Build history of the part. All positions in model axes, mm. A direction names the side the tool comes from. Round coordinates to 2 decimals unless told otherwise and drop trailing zeros. Order: outer loops, then holes, each group sorted by start corner. A loop starts at its lowest first (then second) coordinate and runs counter-clockwise, first axis right, second up. Notation, with made-up numbers: (0, -38.5) -> (31, -38.5) arc R26 ccw to (31, -2.5) -> close; hole circle Ø4 at (-38, 63.25). An arc over 180 degrees is marked (long way). Answer as a JSON object with one key per item and string values.
from build123d import *

# Parameters (mm, degrees)
SKETCH_3_W          = 100
SKETCH_3_H          = 40
EXTRUDE_1_DEPTH     = 10
EXTRUDE_3_DEPTH     = 10
SKETCH_6_R          = 12.5
CUT_EXTRUDE_1_DEPTH = 5
SKETCH_8_R          = 6
CUT_EXTRUDE_2_DEPTH = 5
SKETCH_9_W          = 30
SKETCH_9_H          = 5
CUT_EXTRUDE_4_DEPTH = 85.409715081
FILLET_1_R          = 8
SKETCH_12_R         = 4
CUT_EXTRUDE_6_DEPTH = 71.178344238
FILLET_2_R          = 3


with BuildPart() as part:
    # Эскиз3 → Бобышка-Вытянуть1 (new body)
    with BuildSketch(Plane(origin=(0, 0, 0), x_dir=(1, 0, 0), z_dir=(0, 1, 0))):
        Rectangle(SKETCH_3_W, SKETCH_3_H)
    extrude(amount=EXTRUDE_1_DEPTH)

    # Эскиз4 → Бобышка-Вытянуть3 (add)
    with BuildSketch(Plane(origin=(0, 0, -20), x_dir=(-1, 0, 0), z_dir=(0, 0, -1))):
        with BuildLine():
            Line((-20, 0), (-20, 35))
            ThreePointArc((-20, 35), (0, 55), (20, 35))
            Line((20, 35), (20, 0))
            Line((20, 0), (-20, 0))
        make_face()
    extrude(amount=-EXTRUDE_3_DEPTH)

    # Эскиз6 → Вырез-Вытянуть1 (cut)
    with BuildSketch(Plane(origin=(0, 0, -20), x_dir=(-1, 0, 0), z_dir=(0, 0, -1))):
        with Locations((0, 35)):
            Circle(SKETCH_6_R)
    extrude(amount=-CUT_EXTRUDE_1_DEPTH, mode=Mode.SUBTRACT)

    # Эскиз8 → Вырез-Вытянуть2 (cut)
    with BuildSketch(Plane(origin=(0, 0, -15), x_dir=(-1, 0, 0), z_dir=(0, 0, -1))):
        with Locations((0, 35)):
            Circle(SKETCH_8_R)
    extrude(amount=-CUT_EXTRUDE_2_DEPTH, mode=Mode.SUBTRACT)

    # Эскиз9 → Вырез-Вытянуть4 (cut, through all)
    with BuildSketch(Plane(origin=(0, 0, -20), x_dir=(-1, 0, 0), z_dir=(0, 0, -1))):
        with Locations((0, 2.5)):
            Rectangle(SKETCH_9_W, SKETCH_9_H)
    extrude(amount=-CUT_EXTRUDE_4_DEPTH, mode=Mode.SUBTRACT)

    # Скругление1
    # the kernel refuses this fillet: 8 mm, written as the material it adds along each edge
    with BuildSketch(Plane(origin=(-15, 5, -20), x_dir=(0, -1, 0), z_dir=(0, 0, 1))) as fillet_1_piece_1:
        with BuildLine():
            CenterArc((8, 7.416198487), FILLET_1_R, 180, 67.975687163)
            Line((0, 7.416198487), (0, 0))
            Line((0, 0), (5, 0))
        make_face()
    extrude(amount=40)
    with BuildSketch(Plane(origin=(15, 5, -20), x_dir=(-1, 0, 0), z_dir=(0, 0, 1))) as fillet_1_piece_2:
        with BuildLine():
            CenterArc((7.416198487, 8), FILLET_1_R, 202.024312837, 67.975687163)
            Line((0, 5), (0, 0))
            Line((0, 0), (7.416198487, 0))
        make_face()
    extrude(amount=40)
    # the kernel refuses this fillet: 8 mm, written as the material it takes off along each edge
    with BuildSketch(Plane(origin=(-50, -20, 20), x_dir=(0, 0, -1), z_dir=(0, 1, 0)), Plane(origin=(-50, -20, -20), x_dir=(1, 0, 0), z_dir=(0, 1, 0))) as fillet_1_2_piece_1:
        with BuildLine():
            CenterArc((FILLET_1_R, -FILLET_1_R), FILLET_1_R, 90, 90)
            Line((0, -FILLET_1_R), (0, 0))
            Line((0, 0), (FILLET_1_R, 0))
        make_face()
    extrude(amount=50, mode=Mode.SUBTRACT)
    with BuildSketch(Plane(origin=(50, -20, 20), x_dir=(0, 0, -1), z_dir=(0, 1, 0)), Plane(origin=(50, -20, -20), x_dir=(-1, 0, 0), z_dir=(0, 1, 0))) as fillet_1_2_piece_2:
        with BuildLine():
            CenterArc((FILLET_1_R, FILLET_1_R), FILLET_1_R, 180, 90)
            Line((0, FILLET_1_R), (0, 0))
            Line((0, 0), (FILLET_1_R, 0))
        make_face()
    extrude(amount=50, mode=Mode.SUBTRACT)

    # Эскиз12 → Вырез-Вытянуть6 (cut, through all)
    with BuildSketch(Plane(origin=(0, 10, 0), x_dir=(1, 0, 0), z_dir=(0, 1, 0))):
        with Locations(Location((-42, -12, 0), (0, 0, 270))):
            Circle(SKETCH_12_R)
        with Locations(Location((42, -12, 0), (0, 0, 90))):
            Circle(SKETCH_12_R)
    extrude(amount=-CUT_EXTRUDE_6_DEPTH, mode=Mode.SUBTRACT)

    # Скругление2
    fillet_2_edges = [part.edges().sort_by_distance(p)[0] for p in [
        (31, 10, -20),
        (20, 10, -15),
        (-20, 10, -15),
        (20, 22.5, -20),
        (0, 55, -20),
        (-20, 22.5, -20),
        (-20, 22.5, -10),
        (0, 10, -10),
        (20, 22.5, -10),
        (0, 55, -10),
        (0, 10, 20),
        (-50, 10, 0),
        (-31, 10, -20),
        (50, 10, 0),
        (47.656854249, 10, -17.656854249),
        (47.656854249, 10, 17.656854249),
        (-47.656854249, 10, -17.656854249),
        (-47.656854249, 10, 17.656854249),
    ]]
    fillet(fillet_2_edges, radius=FILLET_2_R)


solid = part.part
1) Probe L1, parallel to X at y = 6, z = 12; L2, parallel to Y at x = 0, z = -13; L3, parallel to Y at x = 4.5, z = -5.5. List the from-to ranges inside material, lowest first. Write a range as from..to.
Checked values:
{"L1": "x = -50..-46, -38..38, 46..50", "L2": "y = 5..29, 41..55", "L3": "y = 5..10"}
2) Pull direction Z, two halves, no side cores. Call faces 1 (the face through (-38.034, 5.07, 11.479)), 2 (the face through (2.71, 22.797, -17.535)), 3 (the face through (38.034, 5.07, 12.521)), 4 (the face through (19.1, 24.15, -19.14)): pulls with the +Z half, pulls with the -Z half, needs draft (parallel to the pull), parting line crosses it, or undercut.
Checked values:
{"face 1": "undercut", "face 2": "needs draft", "face 3": "undercut", "face 4": "pulls with the -Z half"}
3) Cut at D-D, the plane z = 15. Count the separate pieces of the cut face and the enclosed holes in it, plus the area to 3 significant figures.
Checked values:
{"separate pieces": "3", "enclosed holes": "0", "area": "749 mm²"}
4) Cut at A-A, the plane x = 0. Give the cut face in (y, z), plus the area to 3 significant figures.
Checked values:
{"outline": "(5, -20) -> (22.5, -20) -> (22.5, -15) -> (29, -15) -> (29, -10) -> (13, -10) arc R3 cw to (10, -7) -> (10, 17) arc R3 ccw to (7, 20) -> (5, 20) -> close; (41, -15) -> (47.5, -15) -> (47.5, -20) -> (52, -20) arc R3 ccw to (55, -17) -> (55, -13) arc R3 ccw to (52, -10) -> (41, -10) -> close", "area": "461 mm²"}
5) Cut at B-B, the plane z = -0.5. Give the cut face in (x, y).
Checked values:
{"outline": "(-50, 0) -> (-15, 0) arc R8 cw to (-7.58, 5) -> (7.58, 5) arc R8 cw to (15, 0) -> (50, 0) -> (50, 7) arc R3 ccw to (47, 10) -> (-47, 10) arc R3 ccw to (-50, 7) -> close"}
6) Which spindle directions (+Z, -Z, +X, -X, +Y, -Y) get a long thin tool onto all of the face, cutting with end or side? Do faces 5 (the face through (0, 5, 0)), 6 (the face through (-19.1, 23.85, -19.14)), 7 (the face through (0, 28, -10)), 8 (the face through (-20, 24, -15)). Say none if no direction does.
Checked values:
{"face 5": "+Z, -Z, -Y", "face 6": "-Z, -X, +Y", "face 7": "+Z, +X, -X, +Y", "face 8": "+Z, -Z, -X, +Y"}
7) Cut at C-C, the plane y = 26. Give the cut face in (x, z), plus the area to 3 significant figures.
Checked values:
{"outline": "(-20, -17) arc R3 ccw to (-17, -20) -> (-8.67, -20) -> (-8.67, -15) -> (8.67, -15) -> (8.67, -20) -> (17, -20) arc R3 ccw to (20, -17) -> (20, -13) arc R3 ccw to (17, -10) -> (-17, -10) arc R3 ccw to (-20, -13) -> close", "area": "306 mm²"}
8) Flat gauge pins, fed straight in: pin 1 Ø4 at (x, z) = (-5.5, 2) entering from -Y; pin 2 Ø5 at (x, z) = (42, 12) entering from +Y; pin 3 Ø1.5 at (x, z) = (-9.5, 3) entering from -Y; pin 4 Ø15 at (x, y) = (0, 35) entering from +Z. Where does each tip first touch, or does it go through?
Checked values:
{"pin 1": "stops at y = 5", "pin 2": "passes through", "pin 3": "stops at y = 4.54", "pin 4": "stops at z = -10"}
